For this review, take the finished solid that the model builds, in its own axes (mm). A direction names the side the tool comes from. Give positions to 0.01 mm unless a question says otherwise; leave off trailing zeros.
from build123d import *

# Parameters (mm, degrees)
CUT_EXTRUDE_1_DEPTH      = 126.12457566
CUT_EXTRUDE_1_DEPTH_BACK = 126.12457566
SKETCH_3_R               = 8
CUT_EXTRUDE_7_DEPTH      = 132.675249315
CUT_EXTRUDE_7_DEPTH_BACK = 100
SKETCH_4_W               = 8
SKETCH_4_H               = 4.126409889


with BuildPart() as part:
    # 草图2 → 旋转1 (revolve)
    with BuildSketch(Plane.XY, mode=Mode.PRIVATE) as revolve_1_sk:
        Polygon((2, 27.983551403), (0, 26), (0, 16), (2, 14), (50, 14), (52, 16), (52, 26), (50, 27.983551403), (31.96542119, 30.261848535), (31.96542119, 63.974361625), (48, 66), (50, 68), (50, 85.45), (48, 85.45), (45.286294211, 77.568826128), (43.286294211, 77.568826128), (40.556999042, 85.495274844), (35.556999042, 85.495274844), (32.843293253, 77.614100973), (30.843293253, 77.614100973), (28.113998085, 85.540549689), (23.113998085, 85.540549689), (20.400292296, 77.659375817), (18.400292296, 77.614100973), (15.670997127, 85.540549689), (10.670997127, 85.540549689), (7.941701959, 77.614100973), (5.941701959, 77.614100973), (3.212406791, 85.540549689), (2, 85.540549689), (2, 68), (4, 66), (20, 63.978729945), (20, 30.261848535), align=None)
    revolve(revolve_1_sk.sketch.rotate(Axis((0, 0, 0), (1, 0, 0)), 90), axis=Axis((0, 0, 0), (1, 0, 0)))

    # 草图3 → 切除-拉伸1 (cut, two sides: drawn at the far end of the back side and taken through both)
    with BuildSketch(Plane(origin=(31.96542119, 0, 0), x_dir=(0, 0, -1), z_dir=(1, 0, 0)).offset(-CUT_EXTRUDE_1_DEPTH_BACK)):
        with Locations((34.095485037, 34.095485037)):
            Circle(SKETCH_3_R)
        with Locations((0, 48)):
            Circle(SKETCH_3_R)
        with Locations((-33.941125497, 33.941125497)):
            Circle(SKETCH_3_R)
        with Locations((-48, 0)):
            Circle(SKETCH_3_R)
        with Locations((0, -48)):
            Circle(SKETCH_3_R)
        with Locations((48, 0)):
            Circle(SKETCH_3_R)
        with Locations((33.941125497, -33.941125497)):
            Circle(SKETCH_3_R)
        with Locations((-33.941125497, -33.941125497)):
            Circle(SKETCH_3_R)
    extrude(amount=CUT_EXTRUDE_1_DEPTH + CUT_EXTRUDE_1_DEPTH_BACK, mode=Mode.SUBTRACT)

    # 草图4 → 切除-拉伸7 (cut, two sides: drawn at the far end of the back side and taken through both)
    with BuildSketch(Plane(origin=(0, 0, 0), x_dir=(0, 0, -1), z_dir=(1, 0, 0)).offset(-CUT_EXTRUDE_7_DEPTH_BACK)):
        with Locations((0.004765376, 14.936795055)):
            Rectangle(SKETCH_4_W, SKETCH_4_H)
    extrude(amount=CUT_EXTRUDE_7_DEPTH + CUT_EXTRUDE_7_DEPTH_BACK, mode=Mode.SUBTRACT)


solid = part.part
1) Tool access review of faces 1 (the face through (8.074, -23.429, 74.397)), 2 (the face through (26, 17, 0)), 3 (the face through (1.68, -14.31, 0.58)): name each direction out of +Z, -Z, +X, -X, +Y, -Y from which nothing blocks a thin tool from reaching the whole face with its end or side.
Answer sheet:
face 1: none
face 2: +X, -X
face 3: -X
2) Draft analysis for pull direction X (two halves, no side actions). For faces 4 (the face through (25.9, -33.59, -25.95)), 5 (the face through (2, 38, -57)), 6 (the face through (30.673, 76.253, -16.933)), state which applies: +X half, -X half, draft (parallel to the pull), parting line (faces both ways), or undercut.
Answer sheet:
face 4: draft
face 5: -X half
face 6: undercut
3) We need section A-A on z = 0. Count the separate pieces of the cut face and the enclosed holes in it, then the cut area to 3 significant figures.
Answer sheet:
separate pieces: 4
enclosed holes: 0
area: 3,530 mm2
4) Clearance check with flat-ended pins moving along their axes: pin 1 (21 mm diameter, centred on y = -33.94, z = -33.94, fed in from -X); pin 2 (6 mm diameter, centred on x = 8.5, z = 36, fed in from -Y); pin 3 (4 mm diameter, centred on x = 26, y = -13, fed in from -Z). State where each tip first meets the part, or that it passes through.
Answer sheet:
pin 1: stops at x = 20
pin 2: stops at y = -78.52
pin 3: stops at z = -84.83
5) To check wall thickness, follow line 1 (Z direction, x = 19, y = 6); line 2 (Z direction, x = 6.5, y = -23); line 3 (Z direction, x = 15, y = -15.5). State the ranges of each line that lie inside material, in increasing order.
Answer sheet:
line 1: z = -77.4 to -63.82, -29.53 to -12.65, 12.65 to 29.53, 63.82 to 77.4
line 2: z = -74.13 to -61.53, -16.92 to 16.92, 61.53 to 74.13
line 3: z = -84.12 to -62.72, -25.25 to 25.25, 62.72 to 84.12
